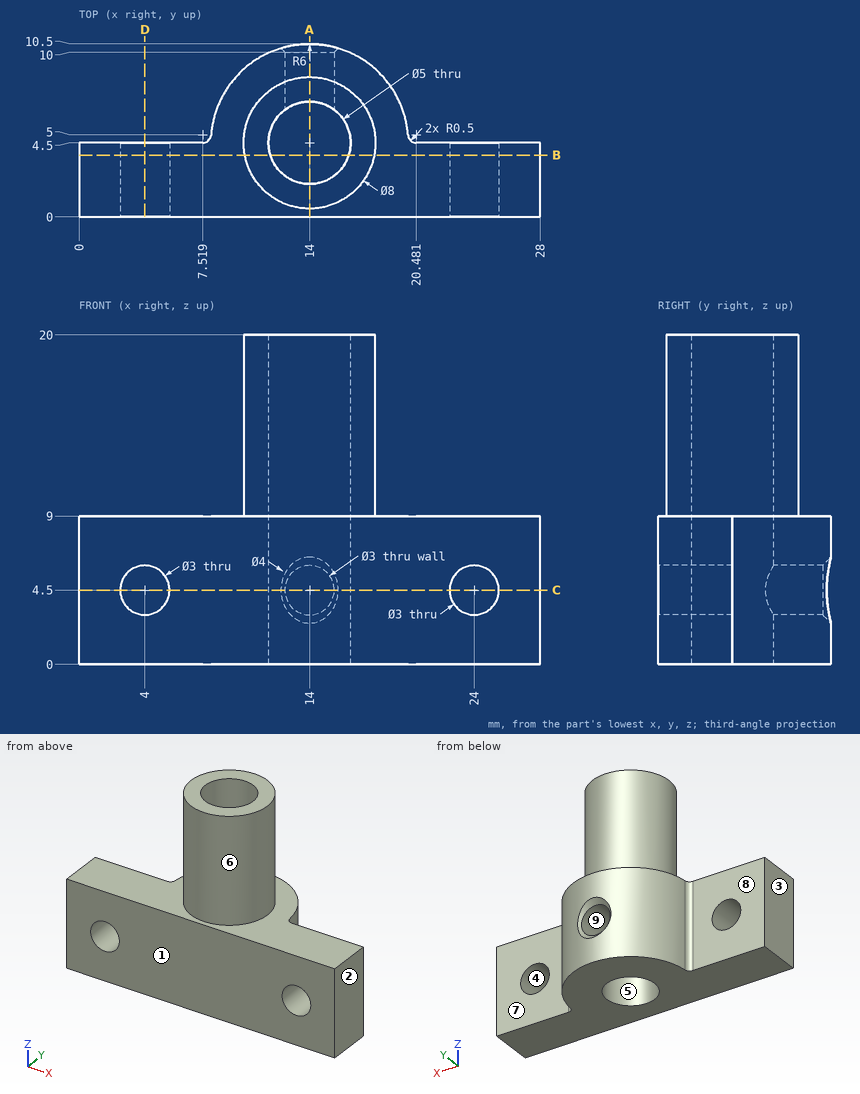
Study the drawing (mm; zero at the part's minimum x, y, z) and answer. A direction names the side the tool comes from. Round coordinates to 2 decimals unless told otherwise and drop trailing zeros. Order: outer loops, then holes, each group sorted by start corner. A loop starts at its lowest first (then second) coordinate and runs counter-clockwise, first axis right, second up. Notation, with made-up numbers: (19.5, 15.25) -> (63.5, 15.25) arc R30 cw to (63.5, 49.25) -> close; hole circle Ø3 at (38, 73). An arc over 180 degrees is marked (long way). Write each question's results on one line, items separated by ' | '. Start each with the question number.
Q1. Each of these flat-tipped pins is pushed along its axis until it touches: pin 1 (5 mm diameter, centred on y = 3.5, z = 15, fed in from -X); pin 2 (1 mm diameter, centred on y = 2, z = 14, fed in from +X); pin 3 (6 mm diameter, centred on x = 4, z = 6, fed in from +Y); pin 4 (5 mm diameter, centred on x = 14, z = 4.5, fed in from +Y). Where does it stop, or does it pass through?
Q2. Straight lines are drawn through the part: probe 1 along X at (y, z) = (1.65, 4.5); probe 2 along Z at (x, y) = (4, 1.95); probe 3 along Y at (x, z) = (14, 12.25). For each, find the intervals that lie inside material, in ascending order. Write a range as from..to.
Q3. Which of the six approach directions +Z, -Z, +X, -X, +Y, -Y give full straight-line access (tool end or side, diameter ignored) to the marked faces 5, 6, 7, 8 and 9?
Q4. Find section D-D (x = 4). Determine the outline of the cut face in (y, z).
Q5. Find section C-C (z = 4.5). Determine the outline of the cut face in (x, y), then the cut area to 3 significant figures.
Q6. The mould has two halves that part along X. Classify the marked faces 1, 2, 3 and 4: pulls with the +X half, pulls with the -X half, needs draft (parallel to the pull), parting line crosses it, or undercut.
Q7. Find section B-B (y = 3.75). Determine the outline of the cut face in (x, z) (1 decimal).
Q8. Find section A-A (x = 14). Determine the outline of the cut face in (y, z).
Worked answers:
1) pin 1: stops at x = 10 | pin 2: stops at x = 17.46 | pin 3: stops at y = 4.5 | pin 4: stops at y = 10.5
2) probe 1: x = 0..2.5, 5.5..22.5, 25.5..28 | probe 2: z = 0..3, 6..9 | probe 3: y = 0.5..2, 7..8.5
3) face 5: +Z, -Z | face 6: +Z | face 7: +Z, -Z, +X, +Y | face 8: +Z, -Z, -X, +Y | face 9: +Y
4) outline: (0, 0) -> (4.5, 0) -> (4.5, 3) -> (0, 3) -> close; (0, 6) -> (4.5, 6) -> (4.5, 9) -> (0, 9) -> close
5) outline: (0, 0) -> (2.5, 0) -> (2.5, 4.5) -> (0, 4.5) -> close; (5.5, 0) -> (22.5, 0) -> (22.5, 4.5) -> (20.48, 4.5) arc R0.5 cw to (19.98, 4.96) arc R6 ccw to (15.74, 10.24) -> (15.5, 10) -> (15.5, 6.5) arc R2.5 cw (long way) to (12.5, 6.5) -> (12.5, 10) -> (12.26, 10.24) arc R6 ccw to (8.02, 4.96) arc R0.5 cw to (7.52, 4.5) -> (5.5, 4.5) -> close; (25.5, 0) -> (28, 0) -> (28, 4.5) -> (25.5, 4.5) -> close | area: 125 mm2
6) face 1: needs draft | face 2: pulls with the +X half | face 3: pulls with the -X half | face 4: undercut
7) outline: (0, 0) -> (11.6, 0) -> (11.6, 20) -> (10.1, 20) -> (10.1, 9) -> (0, 9) -> close; (16.4, 0) -> (28, 0) -> (28, 9) -> (17.9, 9) -> (17.9, 20) -> (16.4, 20) -> close; hole circle Ø3 at (4, 4.5); hole circle Ø3 at (24, 4.5)
8) outline: (0, 0) -> (2, 0) -> (2, 20) -> (0.5, 20) -> (0.5, 9) -> (0, 9) -> close; (7, 0) -> (10.5, 0) -> (10.5, 2.5) -> (10, 3) -> (7, 3) -> close; (7, 6) -> (10, 6) -> (10.5, 6.5) -> (10.5, 9) -> (8.5, 9) -> (8.5, 20) -> (7, 20) -> close
